The figure shows three views and two pictorial views of one solid part (mm, origin at its lowest corner). Answer the questions. A direction names the side the tool comes from. Coordinates: 2 decimals unless noted, no trailing zeros. Write each loop counter-clockwise with the first axis right and the second up, starting at its lowest first coordinate (ties: lowest second). Pieces come first, ordered by that corner, then holes. Notation, with made-up numbers: M -8.75,89 L 18.25,89 A18 cw 18.25,94 Z; hole C 56,38 d4. An arc over 180 degrees is marked long. Write item = value, one per line.
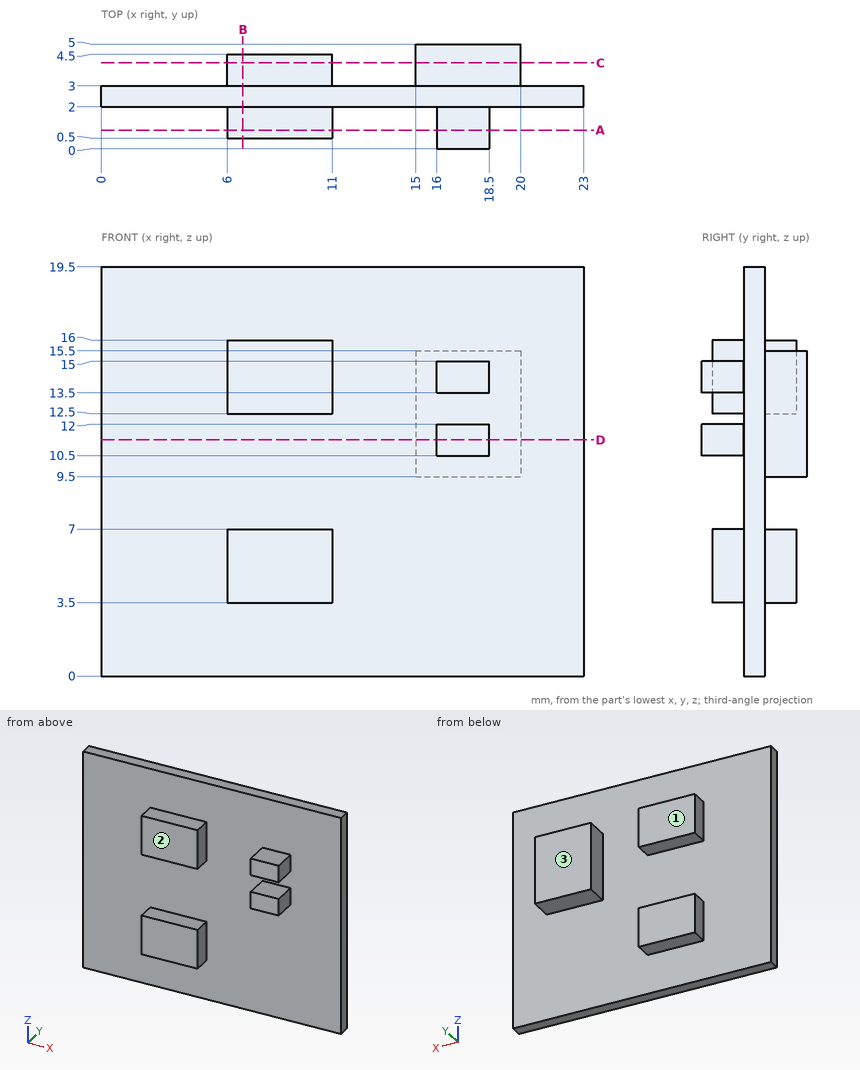
Item 1: Find section C-C (y = 4.1). Determine the outline of the cut face in (x, z), and give its area (3 significant figures).
Worked answers:
outline = M 6,3.5 L 11,3.5 L 11,7 L 6,7 Z; M 6,12.5 L 11,12.5 L 11,16 L 6,16 Z; M 15,9.5 L 20,9.5 L 20,15.5 L 15,15.5 Z
area = 65.0 mm²
Item 2: Find section B-B (x = 6.75). Determine the outline of the cut face in (y, z), and give its area (3 significant figures).
Worked answers:
outline = M 0.5,3.5 L 2,3.5 L 2,0 L 3,0 L 3,3.5 L 4.5,3.5 L 4.5,7 L 3,7 L 3,12.5 L 4.5,12.5 L 4.5,16 L 3,16 L 3,19.5 L 2,19.5 L 2,16 L 0.5,16 L 0.5,12.5 L 2,12.5 L 2,7 L 0.5,7 Z
area = 40.5 mm²
Item 3: Which of the six approach directions +Z, -Z, +X, -X, +Y, -Y give full straight-line access (tool end or side, diameter ignored) to the marked faces 1, 2 and 3?
Worked answers:
face_1 = +Z, -Z, -X, +Y
face_2 = +Z, -Z, -X, -Y
face_3 = +Z, -Z, +X, -X, +Y
Item 4: Flat-ended cylindrical pins translate along their axes: pin 1 (1.2 mm diameter, centred on y = 0.5, z = 11, fed in from +X); pin 2 (4 mm diameter, centred on x = 10.5, z = 14.5, fed in from +Y); pin 3 (1.6 mm diameter, centred on x = 18, y = 4, fed in from +Z). Find the tip coordinate at first contact, or state that the pin passes through.
Worked answers:
pin_1 = 18.5
pin_2 = 4.5
pin_3 = 15.5
Item 5: Consider line 1 along Z through (x, y) = (16.75, 0.4); line 2 along Y through (x, z) = (12, 9.25); line 3 along X through (y, z) = (3.3, 14.5). Determine where each line is inside the solid, lowest interval first. Write a range as from..to.
Worked answers:
line_1 = 10.5..12, 13.5..15
line_2 = 2..3
line_3 = 6..11, 15..20
Item 6: Find section D-D (z = 11.25). Determine the outline of the cut face in (x, y), and give its area (3 significant figures).
Worked answers:
outline = M 0,2 L 16,2 L 16,0 L 18.5,0 L 18.5,2 L 23,2 L 23,3 L 20,3 L 20,5 L 15,5 L 15,3 L 0,3 Z
area = 38.0 mm²
Item 7: Find section A-A (y = 0.9). Determine the outline of the cut face in (x, z), and give its area (3 significant figures).
Worked answers:
outline = M 6,3.5 L 11,3.5 L 11,7 L 6,7 Z; M 6,12.5 L 11,12.5 L 11,16 L 6,16 Z; M 16,10.5 L 18.5,10.5 L 18.5,12 L 16,12 Z; M 16,13.5 L 18.5,13.5 L 18.5,15 L 16,15 Z
area = 42.5 mm²
